Design review of the part built by this model. Coordinates are the model's own, in mm. A direction names the side the tool comes from. Coordinates: 2 decimals unless noted, no trailing zeros. Loops run counter-clockwise (first coordinate to the right, second up) from the corner with the lowest first, then second, coordinate; pieces in that order, holes last. Notation, with made-up numbers: M -31.75,29 L -22.75,29 A21 ccw -22.75,55 Z; hole C 19.25,6 d4. An arc over 180 degrees is marked long. Answer as CSV lines item,"result". Start each with the question number.
from build123d import *

# Parameters (mm, degrees)
SKETCH2_W           = 40
SKETCH2_H           = 40
SKETCH2_W_2         = 36
SKETCH2_H_2         = 36
BOSS_EXTRUDE1_DEPTH = 1631.5
CUT_EXTRUDE1_REACH  = 1897.948


with BuildPart() as part:
    # Sketch2 → Boss-Extrude1 (new body)
    with BuildSketch(Plane(origin=(0, 1631.5, 0), x_dir=(1, 0, 0), z_dir=(0, 1, 0))):
        with Locations((945, 20)):
            Rectangle(SKETCH2_W, SKETCH2_H)
        with Locations((945, 20)):
            Rectangle(SKETCH2_W_2, SKETCH2_H_2, mode=Mode.SUBTRACT)
    extrude(amount=-BOSS_EXTRUDE1_DEPTH)

    # Cut-Extrude1: up to this face of the body (flat: up to its plane)
    cut_extrude1_end = Plane(part.part.faces().sort_by_distance((945, 815.75, -40))[0])
    # Sketch3 → Cut-Extrude1 (cut, up to the picked face)
    with BuildSketch(Plane.XY, mode=Mode.PRIVATE) as cut_extrude1_sk1:
        Polygon((965, 0), (965, 40), (925, 0), align=None)
    cut_extrude1_tool1 = split(extrude(cut_extrude1_sk1.sketch, amount=-CUT_EXTRUDE1_REACH, mode=Mode.PRIVATE), bisect_by=cut_extrude1_end, keep=Keep.BOTH, mode=Mode.PRIVATE)
    # Sketch3 → Cut-Extrude1 (cut, up to the picked face)
    with BuildSketch(Plane.XY, mode=Mode.PRIVATE) as cut_extrude1_sk2:
        Polygon((965, 1631.5), (925, 1631.5), (965, 1591.5), align=None)
    cut_extrude1_tool2 = split(extrude(cut_extrude1_sk2.sketch, amount=-CUT_EXTRUDE1_REACH, mode=Mode.PRIVATE), bisect_by=cut_extrude1_end, keep=Keep.BOTH, mode=Mode.PRIVATE)
    add(cut_extrude1_tool1.solids().sort_by(Axis((951.666667, 13.333333, 0), (0, 0, -1)))[0], mode=Mode.SUBTRACT)
    add(cut_extrude1_tool2.solids().sort_by(Axis((951.666667, 1618.166667, 0), (0, 0, -1)))[0], mode=Mode.SUBTRACT)


solid = part.part
Item 1: Add section C-C (y = 848.5). Give the boundary of the cut face in (x, z), plus the area to 3 significant figures.
Item 2: Mouldability with a two-part tool opening along X and no side actions: class faces 1 (the face through (943.4, 1613.1, -39.2)), 2 (the face through (945, 827, -38)), 3 (the face through (945, 827, -40)) as released by +X, released by -X, zero draft, split by the parting line, or undercut.
Item 3: For pin 1 (3 mm diameter, centred on x = 943, y = 905, fed in from +Z); pin 2 (8 mm diameter, centred on x = 960, z = -21.5, fed in from +Y), all flat-tipped, find the tip position at first contact; note any pin that passes through.
Item 4: Add section A-A (z = -28.5). Give the boundary of the cut face in (x, y), plus the area to 3 significant figures.
Item 5: For line 1 along X through (y, z) = (560, -28); line 2 along Z through (x, y) = (953.5, 183), list the stretches that pass through material, from the lowest coordinate up. Write a range as from..to.
Item 6: Add section B-B (x = 941). Give the boundary of the cut face in (y, z).
Item 7: For faces 4 (the face through (947, 22, -39)), 5 (the face through (945, 827, -2)), list the 3-axis set-ups (+Z, -Z, +X, -X, +Y, -Y) from which the entire face can be reached by the end or side of a thin tool; tool diameter is ignored.
Response:
1,outline,"M 925,-40 L 965,-40 L 965,0 L 925,0 Z; hole M 927,-38 L 963,-38 L 963,-2 L 927,-2 Z"
1,area,"304 mm²"
2,face 1,"released by +X"
2,face 2,"undercut"
2,face 3,"zero draft"
3,pin 1,"z = 0"
3,pin 2,"y = 1593.5"
4,outline,"M 925,0 L 927,2 L 927,1629.5 L 925,1631.5 Z; M 963,38 L 965,40 L 965,1591.5 L 963,1593.5 Z"
4,area,"6,370 mm²"
5,line 1,"925..927, 963..965"
5,line 2,"-40..-38, -2..0"
6,outline,"M 16,-40 L 1615.5,-40 L 1615.5,-38 L 16,-38 Z; M 16,-2 L 1615.5,-2 L 1615.5,0 L 16,0 Z"
7,face 4,"+Z, -Z, +X, -Y"
7,face 5,"+Y, -Y"
